Work out the finished part from the listing and answer in its coordinate system (mm). Face numbers are marked on the shaded views. A direction names the side the tool comes from. Round coordinates to 2 decimals unless told otherwise and drop trailing zeros. Order: outer loops, then holes, each group sorted by start corner. A loop starts at its lowest first (then second) coordinate and runs counter-clockwise, first axis right, second up. Notation, with made-up numbers: (-2.5, 75.25) - (51.5, 75.25) arc R17 cw to (51.5, 87.25) - close; hole circle Ø8 at (35.5, 81.5). An arc over 180 degrees is marked (long way). Use one line per item in the form item = value. Start each with the question number.
Q1. The part is cut by section A-A on x = 14. Determine the outline of the cut face in (y, z), plus the area to 3 significant figures.
Q2. Find the intervals of material crossed by line 1 (Y direction, x = 16.5, z = -1.5); line 2 (Z direction, x = 19.5, y = 1); line 3 (Y direction, x = 6, z = 0.8), in increasing order. Write a range as [from, to].
Q3. Given P1, Ø2, axis at x = 21, z = -0.5, coming from the -Y side; P2, Ø2, axis at x = 9, y = -0.5, coming from the +Z side, each flat-ended and moving along its own axis, determine where each tip first touches the part or whether it passes through.
Q4. Which of the six approach directions +Z, -Z, +X, -X, +Y, -Y give full straight-line access (tool end or side, diameter ignored) to the marked faces 1 and 2?
Q5. The part is cut by section B-B on x = 24.5. Determine the outline of the cut face in (y, z), plus the area to 3 significant figures.
from build123d import *

# Parameters (mm, degrees)
CORTE_EXTRUS_O2_DEPTH = 5
CORTE_EXTRUS_O1_DEPTH = 10


with BuildPart() as part:
    # Esboço1 → Revolução1 (revolve)
    with BuildSketch(Plane.XY, mode=Mode.PRIVATE) as revolu_o1_sk:
        Polygon((6.2, 2.25), (6.2, 1.8), (12.2, 1.8), (12.35, 1.65), (23.1, 1.65), (28.1, 1.05), (28.1, 0), (0, 0), (0, 1.970292752), (4, 2.25), (4.7, 2.25), align=None)
    revolve(revolu_o1_sk.sketch.rotate(Axis((0, 0, 0), (1, 0, 0)), 90), axis=Axis((0, 0, 0), (1, 0, 0)))

    # Esboço2 → Corte-extrusão2 (cut, symmetric)
    with BuildSketch(Plane.XY):
        Polygon((0, 1.970292752), (1.471712801, -2.073204936), (2.326234143, -4.420983029), (-0.931248246, -4.420983029), (-0.931248246, 3.056454726), (-0.395330628, 3.056454726), align=None)
    extrude(amount=CORTE_EXTRUS_O2_DEPTH, both=True, mode=Mode.SUBTRACT)

    # Esboço3 → Corte-extrusão1 (cut, along a direction that is not the sketch's normal)
    with BuildSketch(Plane(origin=(3.863561719, 2.25, 0), x_dir=(0, 0, -1), z_dir=(0, 1, 0))):
        with BuildLine():
            Line((-4.503319596, -3.136438281), (-0.692801568, 3.463572547))
            ThreePointArc((-0.692801568, 3.463572547), (0, 3.863561719), (0.692801568, 3.463572547))
            Line((0.692801568, 3.463572547), (4.503319596, -3.136438281))
            ThreePointArc((4.503319596, -3.136438281), (0, 13.670179255), (-4.503319596, -3.136438281))
        make_face()
    extrude(amount=-CORTE_EXTRUS_O1_DEPTH, dir=(-0.3420201433256694, 0.9396926207859082, 0), mode=Mode.SUBTRACT)


solid = part.part
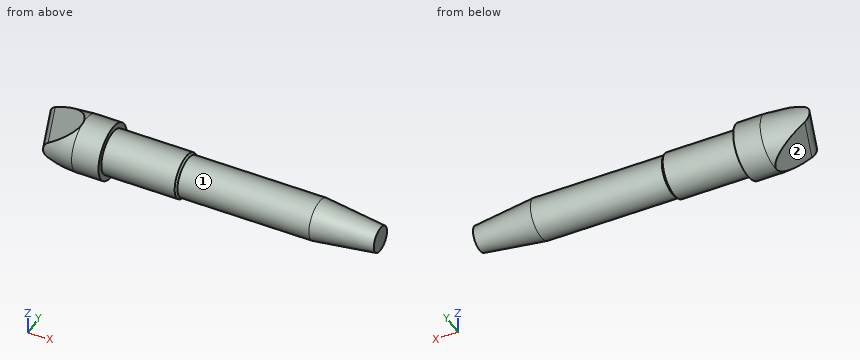
Found:
q1.outline = circle Ø3.3 at (0, 0)
q1.area = 8.55 mm²
q2.line_1 = [-0.69, 0.69]
q2.line_2 = [-1.31, 1.31]
q2.line_3 = [-2.1, 2.1]
q3.P1 = -1.65
q3.P2 = 1.8
q4.face_1 = +X
q4.face_2 = -Z, -X, -Y
q5.outline = circle Ø2.96 at (0, 0)
q5.area = 6.90 mm²
